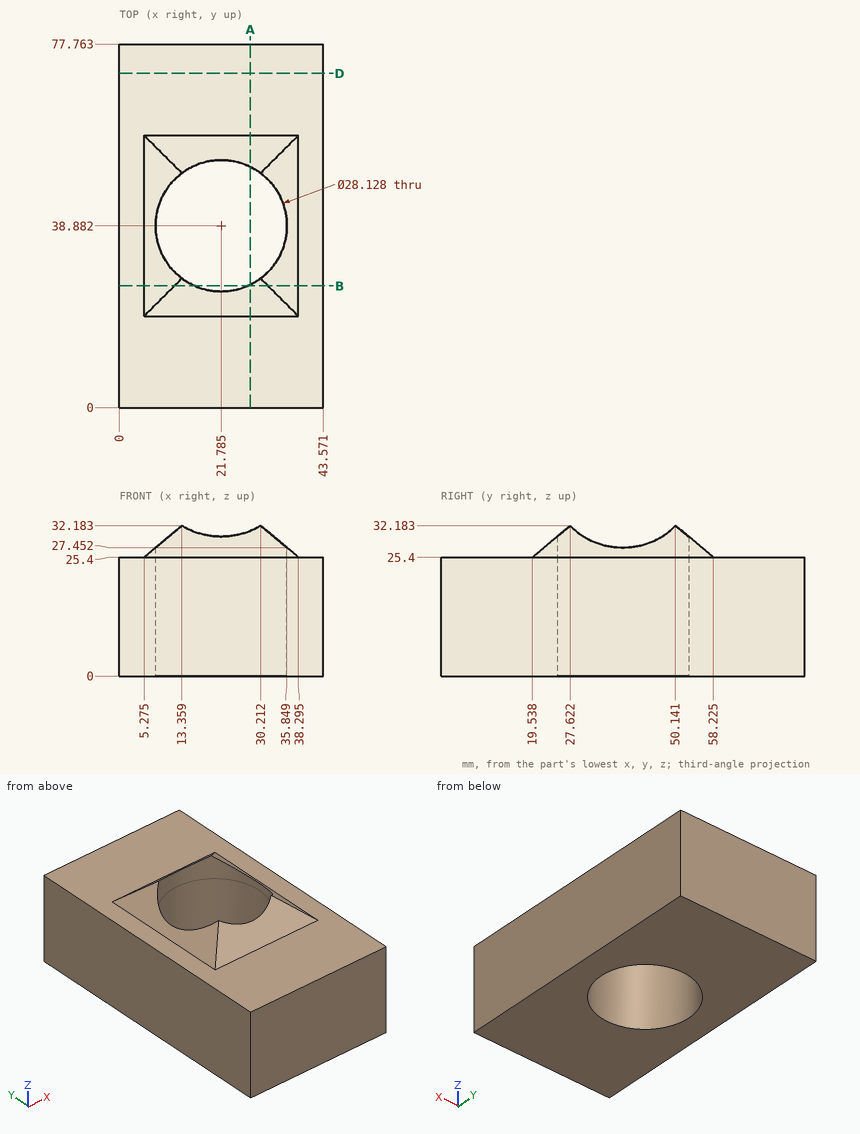
Here's the drawing with two shaded views (mm, measured from the low corner). I have some questions. Round coordinates to 2 decimals unless told otherwise and drop trailing zeros. Loops run counter-clockwise (first coordinate to the right, second up) from the corner with the lowest first, then second, coordinate; pieces in that order, holes last. Notation, with made-up numbers: M 7.5,71 L 45.5,71 A24 cw 45.5,105 Z; hole C -29.75,11.5 d5. An arc over 180 degrees is marked long. Put each result on its own line as item: value.
Q1. Imagine slicing it at B-B (y = 26). Write out the boundary of the cut face in (x, z) (1 decimal), then the cut area to 3 significant figures.
Check result:
outline: M 0,0 L 16.1,0 L 16.1,30.8 L 11.7,30.8 L 5.3,25.4 L 0,25.4 Z; M 27.4,0 L 43.6,0 L 43.6,25.4 L 38.3,25.4 L 31.8,30.8 L 27.4,30.8 Z
area: 903 mm2
Q2. Imagine slicing it at D-D (y = 71.5). Write out the boundary of the cut face in (x, z).
Check result:
outline: M 0,0 L 43.57,0 L 43.57,25.4 L 0,25.4 Z
Q3. I need wall thicknesses on probe 1 along X at (y, z) = (39, 22); probe 2 along Z at (x, y) = (25, 8.5); probe 3 along Y at (x, z) = (29, 27) (1 decimal). Which ranges of each line are inside material? Lowest first, please.
Check result:
probe 1: 0 to 7.72, 35.85 to 43.57
probe 2: 0 to 25.4
probe 3: 21.4 to 26.8, 51 to 56.3
Q4. Imagine slicing it at A-A (x = 28). Write out the boundary of the cut face in (y, z) (1 decimal), then the cut area to 3 significant figures.
Check result:
outline: M 0,0 L 26.3,0 L 26.3,31 L 19.5,25.4 L 0,25.4 Z; M 51.5,0 L 77.8,0 L 77.8,25.4 L 58.2,25.4 L 51.5,31 Z
area: 1,370 mm2
Q5. For pin 1 (6 mm diameter, centred on x = 22.5, y = 25, fed in from +Z) (1 decimal), with a flat end and sliding along its axis, tell me the tip position at first contact or that it passes through.
Check result:
pin 1: z = 30.2
